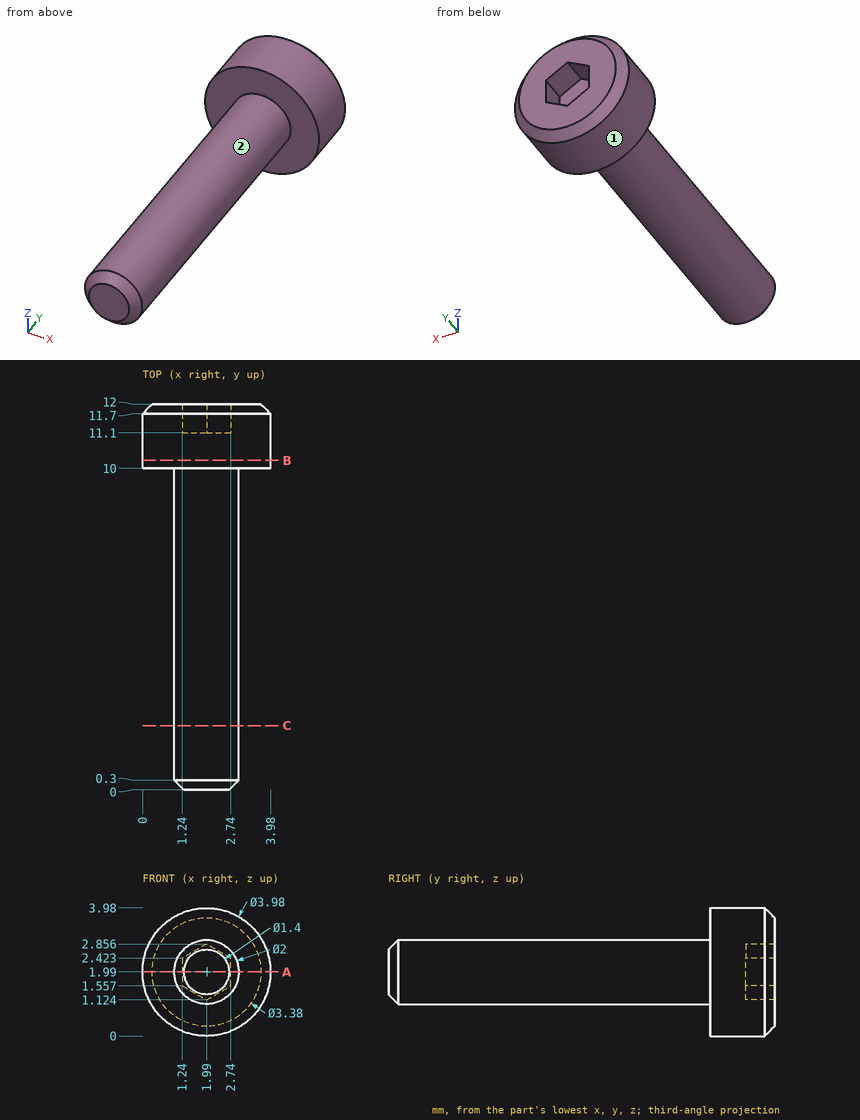
Answer from the drawing. Dimensions are ordinates in mm from the lowest x, y and z of the part. A direction names the side the tool comes from. Give positions to 0.01 mm unless a question says otherwise; leave off trailing zeros. Loops run counter-clockwise (first coordinate to the right, second up) from the corner with the lowest first, then second, coordinate; pieces in that order, holes last.
Item 1: The part is cut by section A-A (z = 1.99). Write down the section's boundary in (x, y).
Item 2: The part is cut by section C-C (y = 2). Write down the section's boundary in (x, z), and give its area (3 significant figures).
Item 3: For the marked faces 1 and 2, determine the directions among +Z, -Z, +X, -X, +Y, -Y from which every point of the face is accessible in a straight line to the end or side of a thin tool.
Item 4: Each of these flat-tipped pins is pushed along its axis until it touches: pin 1 Ø1 at (x, y) = (3, 10) entering from +Z; pin 2 Ø2 at (y, z) = (6.5, 3) entering from +X; pin 3 Ø0.5 at (x, z) = (2, 2) entering from +Y. Where does it stop, or does it pass through?
Item 5: Find the intervals of material crossed by line 1 along Y through (x, z) = (0.7, 1.3); line 2 along X through (y, z) = (5.25, 1.95); line 3 along X through (y, z) = (5.75, 1.25), in increasing order.
Item 6: The part is cut by section B-B (y = 10.25). Write down the section's boundary in (x, z).
Taken from the geometry:
1. outline: (0, 10) - (0.99, 10) - (0.99, 0.3) - (1.29, 0) - (2.69, 0) - (2.99, 0.3) - (2.99, 10) - (3.98, 10) - (3.98, 11.7) - (3.68, 12) - (2.74, 12) - (2.74, 11.1) - (1.24, 11.1) - (1.24, 12) - (0.3, 12) - (0, 11.7) - close
2. outline: circle Ø2 at (1.99, 1.99)
2. area: 3.14 mm2
3. face 1: +Y, -Y
3. face 2: -Y
4. pin 1: stops at z = 3.91
4. pin 2: stops at x = 2.99
4. pin 3: stops at y = 11.1
5. line 1: y = 10 to 12
5. line 2: x = 0.99 to 2.99
5. line 3: x = 1.32 to 2.66
6. outline: circle Ø3.98 at (1.99, 1.99)
